Check sheet for the modelled part. Datum: model origin and axes. Units: mm. A direction names the side the tool comes from. Coordinates: 2 decimals unless noted, no trailing zeros. Write each loop counter-clockwise with the first axis right and the second up, starting at its lowest first coordinate (ties: lowest second). Pieces come first, ordered by that corner, then holes. Notation, with made-up numbers: M 59,2 L 71,2 A27 ccw 71,40 Z; hole C 11,-27.75 d6. An arc over 180 degrees is marked long. Answer as CSV lines item,"result". Start each with the question number.
1) Material ranges on L1, parallel to Z at x = 171.5, y = 123.5; L2, parallel to Y at x = 81.5, z = 2.25; L3, parallel to Y at x = 205, z = 0.45, recorded low to high. Write a range as [from, to].
2) Section check B-B (x = 58.5). Record the cut outline in (y, z), and give its area (3 significant figures).
3) Draft check along Y on faces 3 (the flat face through (214.639, 146.607, 7.395)), 4 (the flat face through (102, 74, 15)), 5 (the flat face through (-1.835, -9.418, 7.395)), 6 (the flat face through (104, 75, 1.5)). Enter one of: +Y half, -Y half, draft (parallel to the pull), parting line (faces both ways), or undercut.
4) Section check C-C (y = 78). Record the cut outline in (x, z), and give its area (3 significant figures).
5) Go/stop test with flat-tipped pins: pin 1 Ø6 at (y, z) = (90.5, 4) entering from +X; pin 2 Ø2.5 at (x, y) = (205, 148) entering from -Z; pin 3 Ø3 at (y, z) = (140, 9) entering from -X; pin 4 Ø4 at (y, z) = (52.5, 10.5) entering from -X. Record where each tip stops, or that it passes through.
6) Access from +Z, -Z, +X, -X, +Y, -Y to the whole of each face (thin tool, end or side, straight path). Record for faces 1 (the flat face through (99.62, 81.17, 7.4)), 2 (the flat face through (100.502, 79.958, 7.584)).
7) Section check A-A (z = 9). Record the cut outline in (x, y).
from build123d import *

# Parameters (mm, degrees)
SKETCH_2_R          = 1.6
EXTRUDE_1_DEPTH     = 15
SKETCH_3_W          = 12
SKETCH_3_H          = 12
CUT_EXTRUDE_1_DEPTH = 275.381172618


with BuildPart() as part:
    # ｽｹｯﾁ2 → ﾎﾞｽ - 押し出し1 (new body)
    with BuildSketch(Plane.XY):
        Polygon((-10.065580607, 1.98345331), (-1.285388486, -10.17829929), (215.065580607, 146.01654669), (206.285388486, 158.17829929), align=None)
        Circle(SKETCH_2_R, mode=Mode.SUBTRACT)
        with Locations((205, 148)):
            Circle(SKETCH_2_R, mode=Mode.SUBTRACT)
    extrude(amount=EXTRUDE_1_DEPTH)

    # ｽｹｯﾁ3 → ｶｯﾄ - 押し出し1 (cut, through all)
    with BuildSketch(Plane(origin=(210.675484547, 152.09742299, 0), x_dir=(0, 0, -1), z_dir=(0.8107835066939648, 0.5853461414180824, 0))):
        with Locations((-7.5, 0)):
            Rectangle(SKETCH_3_W, SKETCH_3_H)
    extrude(amount=-CUT_EXTRUDE_1_DEPTH, mode=Mode.SUBTRACT)


solid = part.part
Results found:
1,L1,"z = [0, 1.5], [13.5, 15]"
1,L2,"y = [49.59, 51.44], [66.24, 68.09]"
1,L3,"y = [138.75, 146.4], [149.6, 157.25]"
2,outline,"M 32.98,0 L 51.48,0 L 51.48,15 L 32.98,15 Z; hole M 34.83,1.5 L 49.63,1.5 L 49.63,13.5 L 34.83,13.5 Z"
2,area,"99.9 mm2"
3,face 3,"+Y half"
3,face 4,"draft"
3,face 5,"-Y half"
3,face 6,"undercut"
4,outline,"M 95.23,0 L 120.85,0 L 120.85,15 L 95.23,15 Z; hole M 97.79,1.5 L 118.29,1.5 L 118.29,13.5 L 97.79,13.5 Z"
4,area,"138 mm2"
5,pin 1,"stops at x = 142.32"
5,pin 2,"passes through"
5,pin 3,"stops at x = 179.03"
5,pin 4,"stops at x = 57.14"
6,face 1,"+Z, -Z, -X, +Y"
6,face 2,"none"
7,outline,"M -10.07,1.98 L -9.19,0.77 L 207.16,156.96 L 206.29,158.18 Z; M -2.16,-8.96 L -1.29,-10.18 L 215.07,146.02 L 214.19,147.23 Z"
